Verification items for the finished model (mm, model axes). A direction names the side the tool comes from. Give positions to 0.01 mm unless a question says otherwise; leave off trailing zeros. Order: outer loops, then holes, each group sorted by start corner. A loop starts at its lowest first (then second) coordinate and runs counter-clockwise, first axis right, second up. Notation, with made-up numbers: (47.5, 17.25) - (81.5, 17.25) arc R31 cw to (81.5, 49.25) - close; hole circle Ø7 at (79, 45). An arc over 180 degrees is marked (long way). Answer as a JSON object with one key per item and string values.
```python
from build123d import *

# Parameters (mm, degrees)
F1_DEPTH = 100


with BuildPart() as f1:
    # F0 (on Top) → F1 (new body)
    with BuildSketch(Plane.XY):
        with BuildLine():
            ThreePointArc((-10, 9.6687327982), (-21.0421802167, -0.1496946047), (-10.8, -10.8))
            Line((-10.8, -10.8), (-10.8, -10))
            ThreePointArc((-10.8, -10), (-20.2415153605, -0.1496405391), (-10, 8.8660766777))
            Line((-10, 8.8660766777), (-10, 9.2266302988))
            Line((-10, 9.2266302988), (-10, 9.6687327982))
        make_face()
        with BuildLine():
            Line((-10.8, -2.9), (-10.8, -10))
            ThreePointArc((-10.8, -10), (-10.3996405391, -9.9915153605), (-10, -9.9660766777))
            Line((-10, -9.9660766777), (-10, -3.1))
            ThreePointArc((-10, -3.1), (-9.9414213562, -2.9585786438), (-9.8, -2.9))
            Line((-9.8, -2.9), (-8, -2.9))
            Line((-8, -2.9), (-8, -2.1))
            Line((-8, -2.1), (-10, -2.1))
            ThreePointArc((-10, -2.1), (-10.5656854249, -2.3343145751), (-10.8, -2.9))
        make_face()
        with BuildLine():
            Line((-10.8, -10), (-10.8, -10.8))
            ThreePointArc((-10.8, -10.8), (-8.7751543269, -10.5980097532), (-6.8301133517, -10))
            Line((-6.8301133517, -10), (-10, -10))
            Line((-10, -10), (-10, -9.9660766777))
            ThreePointArc((-10, -9.9660766777), (-10.3996405391, -9.9915153605), (-10.8, -10))
        make_face()
        with BuildLine():
            Line((-2.1, -10), (-2.1, -8))
            Line((-2.1, -8), (-2.9, -8))
            Line((-2.9, -8), (-2.9, -9.8))
            ThreePointArc((-2.9, -9.8), (-2.9585786438, -9.9414213562), (-3.1, -10))
            Line((-3.1, -10), (-6.8301133517, -10))
            ThreePointArc((-6.8301133517, -10), (-8.7751543269, -10.5980097532), (-10.8, -10.8))
            Line((-10.8, -10.8), (-2.9, -10.8))
            ThreePointArc((-2.9, -10.8), (-2.3343145751, -10.5656854249), (-2.1, -10))
        make_face()
        with BuildLine():
            ThreePointArc((-9.5512689743, 9.6236508111), (-9.8650543244, 9.5262070088), (-10, 9.2266302988))
            ThreePointArc((-10, 9.2266302988), (-9.8995766936, 8.9615759561), (-9.6487309769, 8.8296097806))
            ThreePointArc((-9.6487309769, 8.8296097806), (-9.3349456572, 8.9270536052), (-9.2, 9.2266302988))
            ThreePointArc((-9.2, 9.2266302988), (-9.3004232901, 9.4916846232), (-9.5512689743, 9.6236508111))
        make_face()
        with BuildLine():
            ThreePointArc((-9.5512689743, 9.6236508111), (-9.7753865117, 9.6486600688), (-10, 9.6687327982))
            Line((-10, 9.6687327982), (-10, 9.2266302988))
            ThreePointArc((-10, 9.2266302988), (-9.8650543244, 9.5262070088), (-9.5512689743, 9.6236508111))
        make_face()
        with BuildLine():
            ThreePointArc((-9.6487309769, 8.8296097806), (-9.8995766936, 8.9615759561), (-10, 9.2266302988))
            Line((-10, 9.2266302988), (-10, 8.8660766777))
            ThreePointArc((-10, 8.8660766777), (-9.8241951226, 8.8494842859), (-9.6487309769, 8.8296097806))
        make_face()
    extrude(amount=F1_DEPTH)


solid = f1.part
```
(1) Section check A-A (x = -18.75). Record the cut outline in (y, z), then the cut area to 3 significant figures.
Computed values:
{"outline": "(-7.02, 0) - (-5.66, 0) - (-5.66, 100) - (-7.02, 100) - close; (4.56, 0) - (5.92, 0) - (5.92, 100) - (4.56, 100) - close", "area": "272 mm²"}
(2) Gauge pin test, flat ends, axial feed: pin 1 Ø2 at (x, z) = (-5, 61.5) entering from +Y; pin 2 Ø1.5 at (y, z) = (-2.5, 20) entering from +X; pin 3 Ø0.6 at (x, z) = (-2.5, 41) entering from +Y; pin 4 Ø10 at (x, y) = (-8.5, 4) entering from -Z. Record the tip position at first contact, or that the pin passes through.
Computed values:
{"pin 1": "stops at y = -10", "pin 2": "stops at x = -8", "pin 3": "stops at y = -8", "pin 4": "stops at z = 0"}
(3) Section check B-B (z = 87). Record the cut outline in (x, y).
Computed values:
{"outline": "(-10.8, -10.8) - (-2.9, -10.8) arc R0.8 ccw to (-2.1, -10) - (-2.1, -8) - (-2.9, -8) - (-2.9, -9.8) arc R0.2 cw to (-3.1, -10) - (-10, -10) - (-10, -3.1) arc R0.2 cw to (-9.8, -2.9) - (-8, -2.9) - (-8, -2.1) - (-10, -2.1) arc R0.8 ccw to (-10.8, -2.9) - (-10.8, -10) arc R9.45 cw (long way) to (-9.65, 8.83) arc R0.4 ccw to (-9.55, 9.62) arc R10.25 ccw (long way) to start"}
(4) Section check D-D (y = 6.5). Record the cut outline in (x, z), then the cut area to 3 significant figures.
Computed values:
{"outline": "(-18.24, 0) - (-17.09, 0) - (-17.09, 100) - (-18.24, 100) - close", "area": "115 mm²"}
(5) Material ranges on line 1 along Y through (x, z) = (-9.75, 90); line 2 along Y through (x, z) = (-7.25, 95); line 3 along Y through (x, z) = (-10.5, 17), recorded low to high. Write a range as [from, to].
Computed values:
{"line 1": "y = [-10.8, -10], [-2.9, -2.1], [8.84, 9.65]", "line 2": "y = [-10.8, -10]", "line 3": "y = [-10.8, -2.28], [8.9, 9.7]"}
(6) Release check for a two-part mould opening along X. For faces 1 (the flat face through (-10, -7, 49)), 2 (the flat face through (-2.1, -9, 49)), 3 (the flat face through (-7, -10.8, 49)) record: pulls with the +X half, pulls with the -X half, needs draft (parallel to the pull), parting line crosses it, or undercut.
Computed values:
{"face 1": "undercut", "face 2": "pulls with the +X half", "face 3": "needs draft"}
(7) Section check C-C (y = -0.55). Record the cut outline in (x, z).
Computed values:
{"outline": "(-21.05, 0) - (-20.25, 0) - (-20.25, 100) - (-21.05, 100) - close"}
(8) Access from +Z, -Z, +X, -X, +Y, -Y to the whole of each face (thin tool, end or side, straight path). Record for faces 4 (the flat face through (-10.8, -6, 49)), 5 (the flat face through (-9, -2.1, 49)), 6 (the flat face through (-10.2, -2.8, 100)), 7 (the flat face through (-2.9, -9, 49)).
Computed values:
{"face 4": "+Z, -Z", "face 5": "+Z, -Z, +X", "face 6": "+Z, +X, -X, +Y, -Y", "face 7": "+Z, -Z, +Y"}
